from build123d import *

# Parameters (mm, degrees)
AUFSATZ_LINEAR_AUSTRAGEN1_DEPTH = 4
SCHNITT_LINEAR_AUSTRAGEN1_REACH = 6
SKIZZE2_R                       = 0.5


with BuildPart() as part:
    # Skizze1 → Aufsatz-Linear austragen1 (new body)
    with BuildSketch(Plane.XY):
        with BuildLine():
            Line((26.5, 8.5), (25.493621062, 8.5))
            ThreePointArc((25.493621062, 8.5), (23.25, 6.256378938), (21.006378938, 8.5))
            Line((21.006378938, 8.5), (19, 8.5))
            Line((19, 8.5), (19, 7.5))
            Line((19, 7.5), (15, 7.5))
            Line((15, 7.5), (15, 8.5))
            Line((15, 8.5), (-15, 8.5))
            Line((-15, 8.5), (-15, 7.5))
            Line((-15, 7.5), (-19, 7.5))
            Line((-19, 7.5), (-19, 8.5))
            Line((-19, 8.5), (-21.006378938, 8.5))
            ThreePointArc((-21.006378938, 8.5), (-23.25, 6.256378938), (-25.493621062, 8.5))
            Line((-25.493621062, 8.5), (-26.5, 8.5))
            Line((-26.5, 8.5), (-26.5, -8.5))
            Line((-26.5, -8.5), (-25.493621062, -8.5))
            ThreePointArc((-25.493621062, -8.5), (-23.25, -6.256378938), (-21.006378938, -8.5))
            Line((-21.006378938, -8.5), (-19, -8.5))
            Line((-19, -8.5), (-19, -7.5))
            Line((-19, -7.5), (-15, -7.5))
            Line((-15, -7.5), (-15, -8.5))
            Line((-15, -8.5), (15, -8.5))
            Line((15, -8.5), (15, -7.5))
            Line((15, -7.5), (19, -7.5))
            Line((19, -7.5), (19, -8.5))
            Line((19, -8.5), (21.006378938, -8.5))
            ThreePointArc((21.006378938, -8.5), (23.25, -6.256378938), (25.493621062, -8.5))
            Line((25.493621062, -8.5), (26.5, -8.5))
            Line((26.5, -8.5), (26.5, 8.5))
        make_face()
    extrude(amount=AUFSATZ_LINEAR_AUSTRAGEN1_DEPTH)

    # Skizze2 → Schnitt-Linear austragen1 (cut, up to next)
    with BuildSketch(Plane.XY.offset(4), mode=Mode.PRIVATE) as schnitt_linear_austragen1_sk1:
        with Locations((-10, 0)):
            Circle(SKIZZE2_R)
    schnitt_linear_austragen1_tool1 = extrude(schnitt_linear_austragen1_sk1.sketch, amount=-SCHNITT_LINEAR_AUSTRAGEN1_REACH, mode=Mode.PRIVATE) & part.part
    add(schnitt_linear_austragen1_tool1.solids().sort_by_distance((-10, 0, 4))[0], mode=Mode.SUBTRACT)
    # Skizze2 → Schnitt-Linear austragen1 (cut, up to next)
    with BuildSketch(Plane.XY.offset(4), mode=Mode.PRIVATE) as schnitt_linear_austragen1_sk2:
        with Locations((10, 0)):
            Circle(SKIZZE2_R)
    schnitt_linear_austragen1_tool2 = extrude(schnitt_linear_austragen1_sk2.sketch, amount=-SCHNITT_LINEAR_AUSTRAGEN1_REACH, mode=Mode.PRIVATE) & part.part
    add(schnitt_linear_austragen1_tool2.solids().sort_by_distance((10, 0, 4))[0], mode=Mode.SUBTRACT)


solid = part.part
The model under review builds one solid part; all positions refer to its coordinate system, in mm. A direction names the side the tool comes from. Round coordinates to 2 decimals unless told otherwise and drop trailing zeros. Order: outer loops, then holes, each group sorted by start corner. A loop starts at its lowest first (then second) coordinate and runs counter-clockwise, first axis right, second up. Notation, with made-up numbers: (5, 54.5) - (55, 54.5) arc R25 ccw to (55, 67.5) - close; hole circle Ø9 at (10, -13). An arc over 180 degrees is marked (long way). Use one line per item in the form item = value.
Q1. Add section C-C on z = 3.25. Give the number of separate pieces and of enclosed holes in the cut face, then the cut area to 3 significant figures.
Response values:
separate_pieces = 1
enclosed_holes = 2
area = 852 mm^2
Q2. Add section B-B on y = 0. Give the boundary of the cut face in (x, z).
Response values:
outline = (-26.5, 0) - (-10.5, 0) - (-10.5, 4) - (-26.5, 4) - close; (-9.5, 0) - (9.5, 0) - (9.5, 4) - (-9.5, 4) - close; (10.5, 0) - (26.5, 0) - (26.5, 4) - (10.5, 4) - close
Q3. Tool access review of faces 4 (the flat face through (-19, 8, 2)), 5 (the cylindrical face through (-10.5, 0, 2)), 6 (the flat face through (-19, -8, 2)): name each direction out of +Z, -Z, +X, -X, +Y, -Y from which nothing blocks a thin tool from reaching the whole face with its end or side.
Response values:
face_4 = +Z, -Z, +Y
face_5 = +Z, -Z
face_6 = +Z, -Z, -Y
Q4. Add section A-A on x = 10. Give the boundary of the cut face in (y, z).
Response values:
outline = (-8.5, 0) - (-0.5, 0) - (-0.5, 4) - (-8.5, 4) - close; (0.5, 0) - (8.5, 0) - (8.5, 4) - (0.5, 4) - close
Q5. To check wall thickness, follow line 1 (Y direction, x = 10, z = 2.8); line 2 (X direction, y = -7, z = 2); line 3 (X direction, y = -6.5, z = 2.45). State the ranges of each line that lie inside material, in increasing order.
Response values:
line_1 = -8.5 to -0.5, 0.5 to 8.5
line_2 = -26.5 to -24.92, -21.58 to 21.58, 24.92 to 26.5
line_3 = -26.5 to -24.27, -22.23 to 22.23, 24.27 to 26.5
Q6. Add section D-D on x = 23.25. Give the boundary of the cut face in (y, z).
Response values:
outline = (-6.26, 0) - (6.26, 0) - (6.26, 4) - (-6.26, 4) - close
Q7. Mouldability with a two-part tool opening along X and no side actions: class faces 1 (the flat face through (0, 0, 0)), 2 (the flat face through (26.5, 0, 2)), 3 (the flat face through (-15, -8, 2)) as pulls with the +X half, pulls with the -X half, needs draft (parallel to the pull), parting line crosses it, or undercut.
Response values:
face_1 = needs draft
face_2 = pulls with the +X half
face_3 = undercut
